Build history of the part. All positions in model axes, mm. Face numbers are marked on the shaded views. A direction names the side the tool comes from. Round coordinates to 2 decimals unless told otherwise and drop trailing zeros. Loops run counter-clockwise (first coordinate to the right, second up) from the corner with the lowest first, then second, coordinate; pieces in that order, holes last. Notation, with made-up numbers: (-34.5, 32.5) -> (-8.5, 32.5) arc R11 cw to (-8.5, 44.5) -> close; hole circle Ø11 at (46, 58). An arc over 180 degrees is marked (long way). Put each result on its own line as item: value. Start each with the question number.
Item 1: Cut at B-B, the plane z = 29. List the corners of the cut face in (x, y).
Item 2: Cut at C-C, the plane x = 4. List the corners of the cut face in (y, z), plus the area to 3 significant figures.
Item 3: Cut at A-A, the plane y = 20. List the corners of the cut face in (x, z).
Item 4: Flat gauge pins, fed straight in: pin 1 Ø8 at (y, z) = (14.5, 28) entering from -X; pin 2 Ø3.5 at (x, z) = (-27, 1) entering from -Y; pin 3 Ø2.5 at (x, z) = (-32.5, 1) entering from +Y. Where does each tip first touch, or does it go through?
Item 5: Tool access for the marked faces 4 and 5: list every direction of +Z, -Z, +X, -X, +Y, -Y with a clear straight run to the whole face (end or side of a thin tool).
Item 6: Drill centre lines: probe 1 along X at (y, z) = (23, 32); probe 2 along Z at (x, y) = (-13, 22); probe 3 along X at (y, z) = (34.5, 4.5). Where is each one in solid material? Low to high. Write a range as [from, to].
Item 7: Pull direction Z, two halves, no side cores. Call the marked faces 1, 2 and 3: +Z half, -Z half, draft (parallel to the pull), parting line (faces both ways), or undercut.
Item 8: Cut at D-D, the plane y = 32.5. List the corners of the cut face in (x, z).
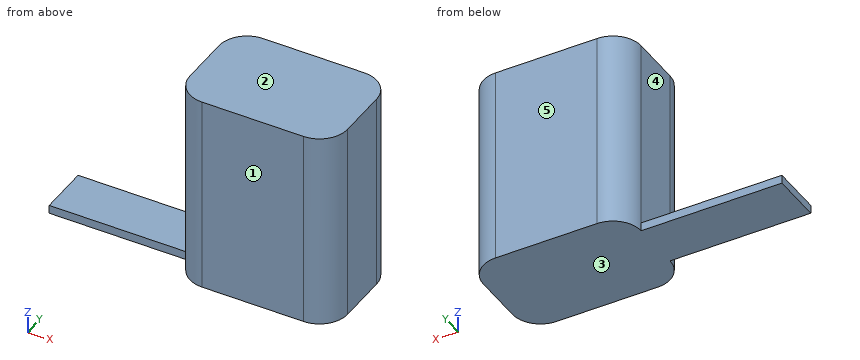
```python
from build123d import *

# Parameters (mm, degrees)
SKETCH_1_W      = 56
SKETCH_1_H      = 38
EXTRUDE_1_DEPTH = 71
FILLET_1_R      = 10
SKETCH_2_W      = 3
SKETCH_2_H      = 18
EXTRUDE_2_DEPTH = 50


with BuildPart() as part:
    # 草图1 → 凸台-拉伸1 (new body)
    with BuildSketch(Plane.XY):
        with Locations((28, 19)):
            Rectangle(SKETCH_1_W, SKETCH_1_H)
    extrude(amount=EXTRUDE_1_DEPTH)

    # 圆角1
    fillet_1_edges = [part.edges().sort_by_distance(p)[0] for p in [
        (0, 38, 35.5),
        (56, 38, 35.5),
        (56, 0, 35.5),
        (0, 0, 35.5),
    ]]
    fillet(fillet_1_edges, radius=FILLET_1_R)

    # 草图2 → 凸台-拉伸2 (add)
    with BuildSketch(Plane.ZY):
        with Locations((1.5, 19)):
            Rectangle(SKETCH_2_W, SKETCH_2_H)
    extrude(amount=EXTRUDE_2_DEPTH)


solid = part.part
```
Reply:
1. outline: (0, 10) arc R10 ccw to (10, 0) -> (46, 0) arc R10 ccw to (56, 10) -> (56, 28) arc R10 ccw to (46, 38) -> (10, 38) arc R10 ccw to (0, 28) -> close
2. outline: (2, 0) -> (36, 0) -> (36, 71) -> (2, 71) -> close
2. area: 2,410 mm^2
3. outline: (-50, 0) -> (56, 0) -> (56, 71) -> (0, 71) -> (0, 3) -> (-50, 3) -> close
4. pin 1: stops at x = 0
4. pin 2: stops at y = 10
4. pin 3: stops at y = 28
5. face 4: +Z, -X, +Y, -Y
5. face 5: +Z, -Z, +X, -X, +Y
6. probe 1: x = [0, 56]
6. probe 2: z = [0, 3]
6. probe 3: x = [2.4, 53.6]
7. face 1: draft
7. face 2: +Z half
7. face 3: -Z half
8. outline: (1.07, 0) -> (54.93, 0) -> (54.93, 71) -> (1.07, 71) -> close
